Could you check a few things on this model? Use its own coordinates, in mm. Face numbers are marked on the shaded views. A direction names the side the tool comes from. Coordinates: 2 decimals unless noted, no trailing zeros. Order: outer loops, then holes, each group sorted by start corner. A loop starts at its lowest first (then second) coordinate and runs counter-clockwise, first axis right, second up. Notation, with made-up numbers: (50.5, 4) -> (90.5, 4) arc R24 cw to (90.5, 42) -> close; hole circle Ø6 at (-16.5, 79.25). An arc over 180 degrees is marked (long way). Use a Markdown table: item, result. Add a question column.
1) Which directions (+Z, -Z, +X, -X, +Y, -Y) give clear straight access to the entire face, cutting with the end or side of a thin tool? Please do the marked faces 1 and 2.
2) Will these pins go through, and if not, where does the flat tip stop? pin 1 Ø1.5 at (x, y) = (0.5, -0.5) entering from +Z; pin 2 Ø0.6 at (x, z) = (0, 0) entering from +Y; pin 3 Ø1 at (x, z) = (-1, 0) entering from -Y.
3) If we section it at D-D (y = -2.25): Write out the boundary of the cut face in (x, z), plus the area to 3 significant figures.
4) If we section it at A-A (z = 0): Write out the boundary of the cut face in (x, y).
5) If we section it at C-C (x = 0): Write out the boundary of the cut face in (y, z).
6) If I drill on L1, parallel to X at y = 2.55, z = 0; L2, parallel to Y at x = 1.1, z = 1.1; L3, parallel to Y at x = -0.6, z = 0.05, over which ranges is the centre line in solid material (lowest first)? Write a range as [from, to].
7) If we section it at B-B (y = 2): Write out the boundary of the cut face in (x, z).
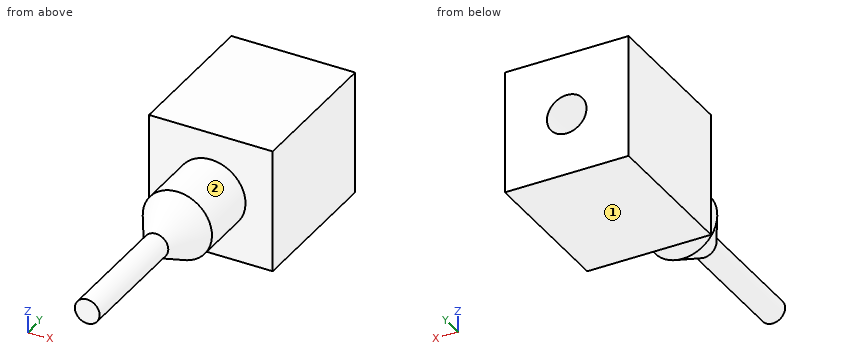
```python
from build123d import *

# Parameters (mm, degrees)
SKETCH_1_W          = 2.5
SKETCH_1_H          = 2.5
EXTRUDE_1_DEPTH     = 3
SKETCH_2_R          = 0.7
EXTRUDE_2_DEPTH     = 2
CHAMFER_1_SIZE      = 0.779422863
CHAMFER_1_SIZE2     = 0.45
SKETCH_3_R          = 0.25
EXTRUDE_3_DEPTH     = 2.5
SKETCH_4_R          = 0.4
CUT_EXTRUDE_1_DEPTH = 2.5


with BuildPart() as part:
    # Эскиз1 → Бобышка-Вытянуть1 (new body)
    with BuildSketch(Plane(origin=(0, 0, 0), x_dir=(1, 0, 0), z_dir=(0, 1, 0))):
        Rectangle(SKETCH_1_W, SKETCH_1_H)
    extrude(amount=EXTRUDE_1_DEPTH)

    # Эскиз2 → Бобышка-Вытянуть2 (add)
    with BuildSketch(Plane.XZ):
        with Locations(Location((0, 0, 0), (0, 0, 270))):
            Circle(SKETCH_2_R)
    extrude(amount=EXTRUDE_2_DEPTH)

    # Фаска1
    chamfer_1_edges = [part.edges().sort_by_distance(p)[0] for p in [
        (0, -2, 0.7),
    ]]
    chamfer_1_side = [part.faces().sort_by_distance(p)[0] for p in [
        (0, -1, 0.7),
    ]]
    chamfer(chamfer_1_edges, length=CHAMFER_1_SIZE, length2=CHAMFER_1_SIZE2, reference=chamfer_1_side[0])

    # Эскиз3 → Бобышка-Вытянуть3 (add)
    with BuildSketch(Plane.XZ.offset(2)):
        with Locations(Location((0, 0, 0), (0, 0, 270))):
            Circle(SKETCH_3_R)
    extrude(amount=EXTRUDE_3_DEPTH)

    # Эскиз4 → Вырез-Вытянуть1 (cut)
    with BuildSketch(Plane(origin=(0, 3, 0), x_dir=(1, 0, 0), z_dir=(0, 1, 0))):
        with Locations(Location((0, 0, 0), (0, 0, 270))):
            Circle(SKETCH_4_R)
    extrude(amount=-CUT_EXTRUDE_1_DEPTH, mode=Mode.SUBTRACT)


solid = part.part
```
Answer sheet:
| question | item | result |
|---|---|---|
| 1 | face 1 | -Z, +X, -X, +Y, -Y |
| 1 | face 2 | -Y |
| 2 | pin 1 | z = 1.25 |
| 2 | pin 2 | y = 0.5 |
| 2 | pin 3 | y = -1.57 |
| 3 | outline | circle Ø0.5 at (0, 0) |
| 3 | area | 0.196 mm2 |
| 4 | outline | (-1.25, 0) -> (-0.7, 0) -> (-0.7, -1.22) -> (-0.25, -2) -> (-0.25, -4.5) -> (0.25, -4.5) -> (0.25, -2) -> (0.7, -1.22) -> (0.7, 0) -> (1.25, 0) -> (1.25, 3) -> (0.4, 3) -> (0.4, 0.5) -> (-0.4, 0.5) -> (-0.4, 3) -> (-1.25, 3) -> close |
| 5 | outline | (-4.5, -0.25) -> (-2, -0.25) -> (-1.22, -0.7) -> (0, -0.7) -> (0, -1.25) -> (3, -1.25) -> (3, -0.4) -> (0.5, -0.4) -> (0.5, 0.4) -> (3, 0.4) -> (3, 1.25) -> (0, 1.25) -> (0, 0.7) -> (-1.22, 0.7) -> (-2, 0.25) -> (-4.5, 0.25) -> close |
| 6 | L1 | [-1.25, -0.4], [0.4, 1.25] |
| 6 | L2 | [0, 3] |
| 6 | L3 | [-1.39, 3] |
| 7 | outline | (-1.25, -1.25) -> (1.25, -1.25) -> (1.25, 1.25) -> (-1.25, 1.25) -> close; hole circle Ø0.8 at (0, 0) |
